from build123d import *

# Parameters (mm, degrees)
WYTNIJ_WYCI_GNI_CIE1_DEPTH      = 5.1
WYTNIJ_WYCI_GNI_CIE1_DEPTH_BACK = 5.1


with BuildPart() as part:
    # Szkic2 → Obrót1 (revolve)
    with BuildSketch(Plane(origin=(0, 0, 0), x_dir=(0, 0, -1), z_dir=(1, 0, 0))):
        Polygon((-3.3, 10.9), (-3.3, 9.9), (-3, 9.9), (-3, 11), (0, 11), (0, 8.6), (-1.35, 8.6), (-1.35, 7.4), (-2.85, 7.4), (-2.85, 1.404592906), (-3.142847868, 0.6), (-3.142847868, 0), (-4.1, 0), (-4.1, 1.5), (-3.4, 1.5), (-3.4, 2.6), (-4.1, 2.6), (-4.1, 10.9), align=None)
    revolve(axis=Axis((0, 0, 0), (0, -1, 0)))

    # Szkic3 → Wytnij-wyciągnięcie1 (cut, two sides)
    with BuildSketch(Plane(origin=(0, 0, 0), x_dir=(0, 0, -1), z_dir=(1, 0, 0))) as wytnij_wyci_gni_cie1_sk:
        with BuildLine():
            Line((-0.4, 0), (-0.4, 6.9))
            ThreePointArc((-0.4, 6.9), (0, 7.3), (0.4, 6.9))
            Line((0.4, 6.9), (0.4, 0))
            Line((0.4, 0), (-0.4, 0))
        make_face()
    extrude(amount=WYTNIJ_WYCI_GNI_CIE1_DEPTH, mode=Mode.SUBTRACT)
    extrude(wytnij_wyci_gni_cie1_sk.sketch, amount=-WYTNIJ_WYCI_GNI_CIE1_DEPTH_BACK, mode=Mode.SUBTRACT)


solid = part.part
For this review, take the finished solid that the model builds, in its own axes (mm). A direction names the side the tool comes from. Coordinates: 2 decimals unless noted, no trailing zeros. Write each loop counter-clockwise with the first axis right and the second up, starting at its lowest first coordinate (ties: lowest second). Pieces come first, ordered by that corner, then holes. Notation, with made-up numbers: (-7.75, -3) -> (42.25, -3) arc R26 cw to (42.25, 32) -> close; hole circle Ø2 at (40.25, 57). An arc over 180 degrees is marked (long way). Write each question's results on one line, items separated by ' | '. Start each with the question number.
1) Consider section D-D (z = 0). Write out the cut boundary in (x, y).
2) Consider section A-A (y = 3.5). Write out the cut boundary in (x, z), plus the area to 3 significant figures.
3) Consider section C-C (y = 10.25). Write out the cut boundary in (x, z).
4) The part is to be moulded in two halves that separate along X. For faces 6 (the face through (-3, 3, -0.4)), 7 (the face through (0, 8.6, 0)), 8 (the face through (0.1, 0.8, 4.1)), say which applies: +X half, -X half, draft (parallel to the pull), parting line (faces both ways), or undercut.
5) For faces 1 (the face through (0.06, 1.26, 2.9)), 2 (the face through (-2.23, 10.39, -2.43)), 3 (the face through (-0.3, 2.6, -3.6)), 4 (the face through (-0.3, 1.5, 3.6)), 5 (the face through (-3, 3, 0.4)), list the 3-axis set-ups (+Z, -Z, +X, -X, +Y, -Y) from which the entire face can be reached by the end or side of a thin tool; tool diameter is ignored.
6) Wall thickness on L1, parallel to X at y = 10.45, z = 0; L2, parallel to Z at x = 0, y = 5.7; L3, parallel to X at y = 7.9, z = 0: over which ranges is each line inside the solid? List them lowest first. Write a range as [from, to].
7) Insertion check: pin 1 (1 mm diameter, centred on x = -3.5, y = 3.5, fed in from -Z); pin 2 (1.4 mm diameter, centred on x = -3.5, y = 2, fed in from +Z); pin 3 (1.5 mm diameter, centred on y = 5, z = 1, fed in from -X). Each pin has a flat end and moves straight along its axis. Give the tip position at first contact, or say it passes through.
Geometry says:
1) outline: (-4.1, 7.3) -> (-2.85, 7.3) -> (-2.85, 7.4) -> (-1.35, 7.4) -> (-1.35, 8.6) -> (1.35, 8.6) -> (1.35, 7.4) -> (2.85, 7.4) -> (2.85, 7.3) -> (4.1, 7.3) -> (4.1, 10.9) -> (3.3, 10.9) -> (3.3, 9.9) -> (3, 9.9) -> (3, 11) -> (-3, 11) -> (-3, 9.9) -> (-3.3, 9.9) -> (-3.3, 10.9) -> (-4.1, 10.9) -> close
2) outline: (-4.08, -0.4) arc R4.1 ccw to (4.08, -0.4) -> (2.82, -0.4) arc R2.85 cw to (-2.82, -0.4) -> close; (-4.08, 0.4) -> (-2.82, 0.4) arc R2.85 cw to (2.82, 0.4) -> (4.08, 0.4) arc R4.1 ccw to start | area: 25.3 mm^2
3) outline: circle Ø8.2 at (0, 0); circle Ø6 at (0, 0); hole circle Ø6.6 at (0, 0)
4) face 6: draft | face 7: undercut | face 8: parting line
5) face 1: -Y | face 2: +Y | face 3: -Z | face 4: +Z | face 5: +X, -X, -Y
6) L1: [-4.1, -3.3], [-3, 3], [3.3, 4.1] | L2: [-4.1, -2.85], [2.85, 4.1] | L3: [-4.1, -1.35], [1.35, 4.1]
7) pin 1: z = -2.79 | pin 2: z = 2.78 | pin 3: x = -4.08
